Design review of the part built by this model. Coordinates are the model's own, in mm. Round coordinates to 2 decimals unless told otherwise and drop trailing zeros. Write each loop counter-clockwise with the first axis right and the second up, starting at its lowest first coordinate (ties: lowest second). Pieces come first, ordered by that corner, then holes. Notation, with made-up numbers: (-4.75, 75) - (27.25, 75) arc R30 ccw to (27.25, 106) - close; hole circle Ø10 at (-17.75, 47.5). An arc over 180 degrees is marked (long way). Use one line per item in the form item = value.
Autodesk Inventor part; units mm, degrees
ref_plane "YZ Plane" through (0, 0, 0) normal (1, 0, 0) x (0, 1, 0)
ref_plane "XZ Plane" through (0, 0, 0) normal (0, 1, 0) x (-1, 0, 0)
ref_plane "XY Plane" through (0, 0, 0) normal (0, 0, 1) x (1, 0, 0)
sketch "Sketch1" plane through (0, 0, 0) normal (0, 1, 0) x (-1, 0, 0)
  line L0 (0, 3.4641) -> (3, 1.7321)
  line L1 (3, 1.7321) -> (3, -1.7321)
  line L2 (3, -1.7321) -> (0, -3.4641)
  line L3 (0, -3.4641) -> (-3, -1.7321)
  line L4 (-3, -1.7321) -> (-3, 1.7321)
  line L5 (-3, 1.7321) -> (0, 3.4641)
  circle A0 centre (0, 0) radius 1.5
  line L6 (0, -4.8497) -> (0, 4.8497)
  dimension "d0" = 3
  dimension "d1" = 6
extrude "Extrusion1" add sketch "Sketch1" along normal blind 5.1 contours L6 A0 L3 L4 L5 | L0 L1 L2 L6 A0
thread "Thread1"
properties part number "Spacer" material "Steel, Mild"
Q1. We need section B-B on z = 0. Write out the cut boundary in (x, y), then the cut area to 3 significant figures.
Calculated:
outline = (-3, 0) - (-1.5, 0) - (-1.5, 5.1) - (-3, 5.1) - close; (1.5, 0) - (3, 0) - (3, 5.1) - (1.5, 5.1) - close
area = 15.3 mm2
Q2. To check wall thickness, follow line 1 along X through (y, z) = (2.6, 0); line 2 along Z through (x, y) = (0.25, 3.1); line 3 along X through (y, z) = (2.35, -1.25). State the ranges of each line that lie inside material, in increasing order. Write a range as from..to.
Calculated:
line_1 = -3..-1.5, 1.5..3
line_2 = -3.32..-1.48, 1.48..3.32
line_3 = -3..-0.83, 0.83..3
Q3. For P1, Ø1.5, axis at x = -1.5, y = 4.5, coming from the -Z side, flat-tipped, find the tip position at first contact; note if it passes through.
Calculated:
P1 = -3.03
Q4. We need section D-D on z = 2. Write out the cut boundary in (x, y), then the cut area to 3 significant figures.
Calculated:
outline = (-2.54, 0) - (2.54, 0) - (2.54, 5.1) - (-2.54, 5.1) - close
area = 25.9 mm2
Q5. We need section C-C on x = -1.15. Write out the cut boundary in (y, z), then the cut area to 3 significant figures.
Calculated:
outline = (0, -2.8) - (5.1, -2.8) - (5.1, -0.96) - (0, -0.96) - close; (0, 0.96) - (5.1, 0.96) - (5.1, 2.8) - (0, 2.8) - close
area = 18.7 mm2
Q6. We need section A-A on y = 3.45. Write out the cut boundary in (x, z), then the cut area to 3 significant figures.
Calculated:
outline = (-3, -1.73) - (0, -3.46) - (3, -1.73) - (3, 1.73) - (0, 3.46) - (-3, 1.73) - close; hole circle Ø3 at (0, 0)
area = 24.1 mm2
Q7. Draft analysis for pull direction Z (two halves, no side actions). For faces 1 (the flat face through (-3, 3, 0)), 2 (the cylindrical face through (1.5, 2.51, -0.07)), 3 (the flat face through (-1.5, 2.5, -2.6)), state which applies: released by +Z, released by -Z, zero draft, split by the parting line, or undercut.
Calculated:
face_1 = zero draft
face_2 = undercut
face_3 = released by -Z
